The model under review builds one solid part; all positions refer to its coordinate system, in mm. Face numbers are marked on the shaded views. Coordinates: 2 decimals unless noted, no trailing zeros. Write each loop counter-clockwise with the first axis right and the second up, starting at its lowest first coordinate (ties: lowest second). Pieces come first, ordered by that corner, then holes.
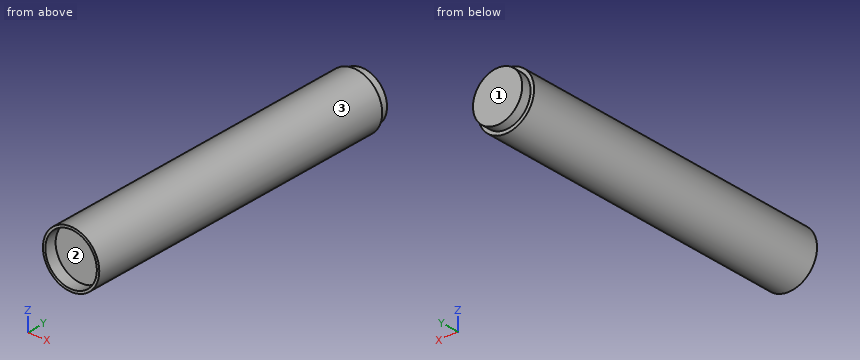
```python
from build123d import *

# Parameters (mm, degrees)
F0_R      = 19.397954
F1_DEPTH  = 223.774
F2_R      = 16.963017
F3_DEPTH  = 6.604
F1_FACE_R = 19.397954
F4_DEPTH  = 5.08
F5_R      = 17.739386
F6_DEPTH  = 8.128


with BuildPart() as f1:
    # F0 (on Front) → F1 (new body)
    with BuildSketch(Plane.XZ):
        Circle(F0_R)
    extrude(amount=F1_DEPTH)

    # F2 (on face) → F3 (join)
    with BuildSketch(Plane(origin=(0, 0, 0), x_dir=(-1, 0, 0), z_dir=(0, 1, 0))):
        Circle(F2_R)
    extrude(amount=F3_DEPTH)

    # F1_face (on face) → F4 (join)
    with BuildSketch(Plane(origin=(0, 0, 0), x_dir=(1, 0, 0), z_dir=(0, 1, 0))):
        Circle(F1_FACE_R)
    extrude(amount=-F4_DEPTH)

    # F5 (on face) → F6 (cut)
    with BuildSketch(Plane.XZ.offset(223.774)):
        Circle(F5_R)
    extrude(amount=-F6_DEPTH, mode=Mode.SUBTRACT)


solid = f1.part
```
Item 1: Mouldability with a two-part tool opening along Z and no side actions: class the marked faces 1, 2 and 3 as pulls with the +Z half, pulls with the -Z half, needs draft (parallel to the pull), parting line crosses it, or undercut.
Solved:
face 1: needs draft
face 2: undercut
face 3: parting line crosses it
Item 2: For pin 1 (4 mm diameter, centred on y = -63.5, z = 1, fed in from -X); pin 2 (4 mm diameter, centred on y = -55, z = 12, fed in from -X); pin 3 (10.5 mm diameter, centred on x = -8, z = -5.5, fed in from -Y); pin 4 (12 mm diameter, centred on y = -43, z = 14, fed in from +X), all flat-tipped, find the tip position at first contact; note any pin that passes through.
Solved:
pin 1: stops at x = -19.4
pin 2: stops at x = -16.62
pin 3: stops at y = -215.65
pin 4: stops at x = 17.67
Item 3: Take a section at C-C, the plane y = -88. Write out the cut boundary in (x, z), plus the area to 3 significant figures.
Solved:
outline: circle Ø38.8 at (0, 0)
area: 1,180 mm2
Item 4: To check wall thickness, follow line 1 along Z through (x, y) = (0, -217); line 2 along Y through (x, z) = (15, 12); line 3 along Y through (x, z) = (6.5, 15). State the ranges of each line that lie inside material, in increasing order.
Solved:
line 1: z = -19.4 to -17.74, 17.74 to 19.4
line 2: y = -223.77 to 0
line 3: y = -215.65 to 6.6
Item 5: Take a section at B-B, the plane z = 0. Write out the cut boundary in (x, y).
Solved:
outline: (-19.4, -223.77) - (-17.74, -223.77) - (-17.74, -215.65) - (17.74, -215.65) - (17.74, -223.77) - (19.4, -223.77) - (19.4, 0) - (16.96, 0) - (16.96, 6.6) - (-16.96, 6.6) - (-16.96, 0) - (-19.4, 0) - close
Item 6: Take a section at A-A, the plane x = 0. Write out the cut boundary in (y, z).
Solved:
outline: (-223.77, -19.4) - (0, -19.4) - (0, -16.96) - (6.6, -16.96) - (6.6, 16.96) - (0, 16.96) - (0, 19.4) - (-223.77, 19.4) - (-223.77, 17.74) - (-215.65, 17.74) - (-215.65, -17.74) - (-223.77, -17.74) - close
